The model under review builds one solid part; all positions refer to its coordinate system, in mm. Face numbers are marked on the shaded views. A direction names the side the tool comes from. Coordinates: 2 decimals unless noted, no trailing zeros. Loops run counter-clockwise (first coordinate to the right, second up) from the corner with the lowest first, then second, coordinate; pieces in that order, holes last. Notation, with made-up numbers: M 48,32 L 57,32 A24 ccw 57,67 Z; hole C 60,68.25 d5. An arc over 180 degrees is marked long. Return JSON: item names as keys, results as strings.
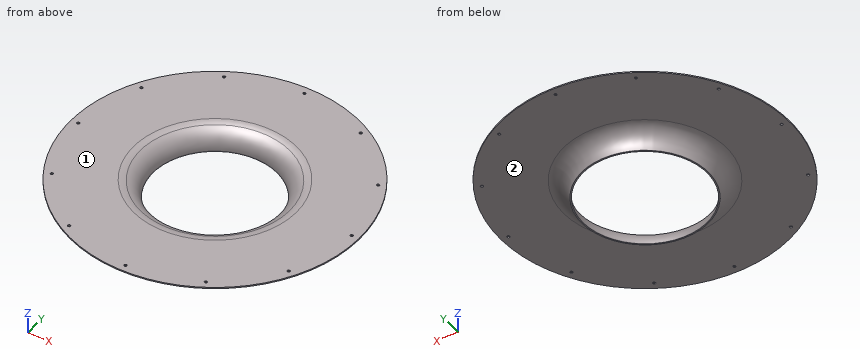
```python
from build123d import *

# Parameters (mm, degrees)
SKETCH1_R          = 357
BASE_FLANGE1_DEPTH = 3
SKETCH2_R          = 156
CUT_EXTRUDE1_DEPTH = 10
CIRPATTERN1_COUNT  = 12


# Read off the part's stored shape, not the designer's step: Edge-Flange1
# Sheet-metal steps are written as plain solids
with BuildPart() as part:
    # Sketch1 → Base-Flange1 (new body)
    with BuildSketch(Plane.XY):
        Circle(SKETCH1_R)
    extrude(amount=-BASE_FLANGE1_DEPTH)

    # Sketch2 → Cut-Extrude1 (cut)
    with BuildSketch(Plane(origin=(0, 0, -3), x_dir=(-1, 0, 0), z_dir=(0, 0, -1))):
        Circle(SKETCH2_R)
    extrude(amount=-CUT_EXTRUDE1_DEPTH, mode=Mode.SUBTRACT)

    # Edge-Flange1 outline → Edge-Flange1 (revolve, cut)
    with BuildSketch(Plane.XZ):
        with BuildLine():
            Line((156, -3), (184.296706911, -3))
            ThreePointArc((184.296706911, -3), (192.514718626, -0.755952756), (201, 0))
            Line((201, 0), (156, 0))
            Line((156, 0), (156, -3))
        make_face()
    revolve(axis=Axis((0, 0, 0), (0, 0, 1)), mode=Mode.SUBTRACT)

    # Edge-Flange1 2 outline → Edge-Flange1 2 (revolve)
    with BuildSketch(Plane.XZ):
        with BuildLine():
            Line((153, -48), (153, -49))
            Line((153, -49), (156, -49))
            Line((156, -49), (156, -48))
            ThreePointArc((156, -48), (169.180194847, -16.180194847), (201, -3))
            Line((201, -3), (184.296706911, -3))
            ThreePointArc((184.296706911, -3), (161.593413823, -20.593413823), (153, -48))
        make_face()
    revolve(axis=Axis((0, 0, 0), (0, 0, 1)))

    # Sketch10 → M8x1.0 Tapped Hole1 (revolve, cut)
    with BuildSketch(Plane(origin=(-339, 0, -3), x_dir=(0, 1, 0), z_dir=(1, 0, 0))):
        Polygon((0, 0), (0, 21.103012167), (3.5, 19), (3.5, 0), align=None)
    m8x1_0_tapped_hole1 = revolve(axis=Axis((-339, 0, -9.35), (0, 0, 1)), mode=Mode.SUBTRACT)

    # CirPattern1: M8x1.0 Tapped Hole1 ×12 about axis
    cirpattern1_axis = Axis((0, 0, 0), (0, 0, 1))
    for i in range(1, CIRPATTERN1_COUNT):
        add(m8x1_0_tapped_hole1.rotate(cirpattern1_axis, i * 360 / CIRPATTERN1_COUNT), mode=Mode.SUBTRACT)


solid = part.part
```
1. Add section B-B on y = 238. Give the boundary of the cut face in (x, z).
Check values:
{"outline": "M -266.09,-3 L 266.09,-3 L 266.09,0 L -266.09,0 Z"}
2. Add section A-A on z = -13. Give the boundary of the cut face in (x, y), plus the area to 3 significant figures.
Check values:
{"outline": "C 0,0 d345.43; hole C 0,0 d336.3", "area": "4,890 mm²"}
3. To check wall thickness, follow line 1 (Y direction, x = 0, z = -48.25); line 2 (Z direction, x = 220, y = 274); line 3 (X direction, y = 91, z = -10). State the ranges of each line that lie inside material, in increasing order.
Check values:
{"line 1": "-156 to -153, 153 to 156", "line 2": "-3 to 0", "line 3": "-151.69 to -145.57, 145.57 to 151.69"}
4. Machinability: for the marked faces 1 and 2, which of the approach directions +Z, -Z, +X, -X, +Y, -Y give a long, thin tool a straight path to every point of the face, cutting with its end or side? Answer none if there is none.
Check values:
{"face 1": "+Z, +X, -X, +Y, -Y", "face 2": "-Z"}
5. Insertion check: pin 1 Ø4 at (x, y) = (169.5, 293.58) entering from +Z; pin 2 Ø1.5 at (x, y) = (42.5, 222) entering from -Z; pin 3 Ø12 at (y, z) = (-73.5, -28) entering from +X. Each pin has a flat end and moves straight along its axis. Give the tip position at first contact, or say it passes through.
Check values:
{"pin 1": "through", "pin 2": "z = -3", "pin 3": "x = 147.76"}
6. Add section C-C on x = -246. Give the boundary of the cut face in (y, z), plus the area to 3 significant figures.
Check values:
{"outline": "M -258.71,-3 L 258.71,-3 L 258.71,0 L -258.71,0 Z", "area": "1,550 mm²"}
